Source: CAD feature listing. Evaluate the final solid. Frame: model axes, mm. Give positions to 0.01 mm unless a question says otherwise; leave off trailing zeros. Loops run counter-clockwise (first coordinate to the right, second up) from the corner with the lowest first, then second, coordinate; pieces in that order, holes last. Notation, with made-up numbers: (49.5, 5.5) -> (58.5, 5.5) arc R18 cw to (58.5, 36.5) -> close; hole circle Ø9 at (-25.75, -36). An arc over 180 degrees is marked (long way). Put each result on its own line as item: value.
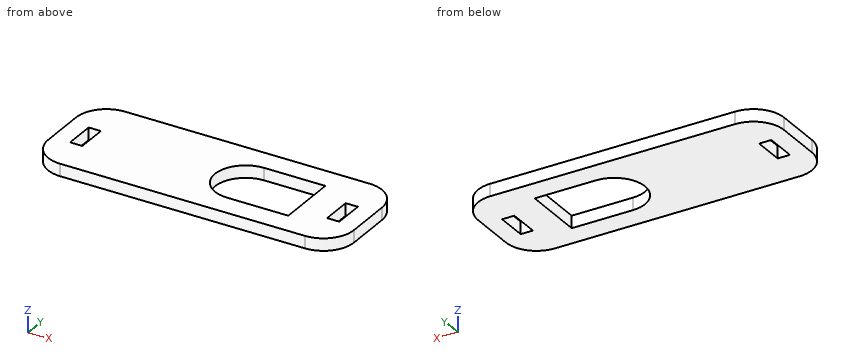
Autodesk Inventor part; units mm, degrees
ref_plane "YZ Plane" through (0, 0, 0) normal (1, 0, 0) x (0, 1, 0)
ref_plane "XZ Plane" through (0, 0, 0) normal (0, 1, 0) x (-1, 0, 0)
ref_plane "XY Plane" through (0, 0, 0) normal (0, 0, 1) x (1, 0, 0)
sketch "Эскиз1" plane through (0, 0, 0) normal (0, 0, 1) x (1, 0, 0)
  line L0 (40, -17.5) -> (22.4906, -17.5)
  arc A0 (40, -17.5) -> (50, -7.5) centre (40, -7.5) ccw
  line L1 (50, 7.5) -> (50, -7.5)
  arc A1 (50, 7.5) -> (40, 17.5) centre (40, 7.5) ccw
  line L2 (22.4906, 17.5) -> (40, 17.5)
  arc A2 (22.4906, 17.5) -> (53.3569, 60.2081) centre (-76.5583, 121.5932) ccw
  arc A3 (53.3569, 60.2081) -> (49.04, 63.7734) centre (57.3118, 69.3928) ccw
  arc A4 (49.04, 63.7734) -> (8.22, 17.5) centre (133.8701, -52.2004) ccw
  line L3 (-8.22, 17.5) -> (8.22, 17.5)
  arc A5 (-8.22, 17.5) -> (-49.04, 63.7734) centre (-133.8701, -52.2004) ccw
  arc A6 (-49.04, 63.7734) -> (-53.3569, 60.2081) centre (-57.3118, 69.3928) ccw
  arc A7 (-53.3569, 60.2081) -> (-22.4906, 17.5) centre (76.5583, 121.5932) ccw
  line L4 (-40, 17.5) -> (-22.4906, 17.5)
  arc A8 (-40, 17.5) -> (-50, 7.5) centre (-40, 7.5) ccw
  line L5 (-50, -7.5) -> (-50, 7.5)
  arc A9 (-50, -7.5) -> (-40, -17.5) centre (-40, -7.5) ccw
  line L6 (-22.4906, -17.5) -> (-40, -17.5)
  arc A10 (-22.4906, -17.5) -> (-53.3569, -60.2081) centre (76.5583, -121.5932) ccw
  arc A11 (-53.3569, -60.2081) -> (-49.04, -63.7734) centre (-57.3118, -69.3928) ccw
  arc A12 (-49.04, -63.7734) -> (-8.22, -17.5) centre (-133.8701, 52.2004) ccw
  line L7 (8.22, -17.5) -> (-8.22, -17.5)
  arc A13 (8.22, -17.5) -> (49.04, -63.7734) centre (133.8701, 52.2004) ccw
  arc A14 (49.04, -63.7734) -> (53.3569, -60.2081) centre (57.3118, -69.3928) ccw
  arc A15 (53.3569, -60.2081) -> (22.4906, -17.5) centre (-76.5583, -121.5932) ccw
  line L8 (22.4906, 17.5) -> (-22.4906, 17.5)
  line L9 (-22.4906, -17.5) -> (22.4906, -17.5)
  line L10 (25, 12.5) -> (25, 8.5)
  line L11 (25, 8.5) -> (15, 8.5)
  line L12 (15, 8.5) -> (15, 12.5)
  line L13 (15, 12.5) -> (25, 12.5)
  line L14 (-15, -8.5) -> (-15, -12.5)
  line L15 (-15, -12.5) -> (-25, -12.5)
  line L16 (-25, -12.5) -> (-25, -8.5)
  line L17 (-25, -8.5) -> (-15, -8.5)
  line L18 (25, -12.5) -> (15, -12.5)
  line L19 (15, -12.5) -> (15, -8.5)
  line L20 (15, -8.5) -> (25, -8.5)
  line L21 (25, -8.5) -> (25, -12.5)
  line L22 (-15, 8.5) -> (-25, 8.5)
  line L23 (-25, 8.5) -> (-25, 12.5)
  line L24 (-25, 12.5) -> (-15, 12.5)
  line L25 (-15, 12.5) -> (-15, 8.5)
  point P0 (0, 0)
  point P1 (8.22, 17.5)
  point P2 (-8.22, -17.5)
extrude "Выдавливание1" add sketch "Эскиз1" along normal blind 4 contours L0 L9 L7 L6 A9 L5 A8 L4 L8 L3 L2 A1 L1 A0 | L10 L11 L12 L13 | L14 L15 L16 L17 | L18 L19 L20 L21 | L22 L23 L24 L25
sketch "Эскиз3" plane through (0, 0, 0) normal (0, 0, -1) x (-1, 0, 0)
  point P0 (0, 0)
sketch "Эскиз4" plane through (0, 0, 0) normal (0, 0, -1) x (-1, 0, 0)
  point P0 (0, 0)
sketch "Эскиз5" plane through (0, 0, 0) normal (0, 0, -1) x (-1, 0, 0)
  line L0 (44, 4.453) -> (44, -5.547)
  line L1 (40, -5.547) -> (40, 4.453)
  line L2 (40, 4.453) -> (44, 4.453)
  line L3 (44, -5.547) -> (40, -5.547)
  line L4 (-44, -5.547) -> (-44, 4.453)
  line L5 (-40, 4.453) -> (-40, -5.547)
  line L6 (-44, 4.453) -> (-40, 4.453)
  line L7 (-40, -5.547) -> (-44, -5.547)
  line L8 (-10, 10) -> (-30, 10)
  line L9 (-30, 10) -> (-30, -10)
  line L10 (-30, -10) -> (-10, -10)
  line L11 (0, 0) -> (0, 0)
  arc A0 (0, 0) -> (-10, 10) centre (-10, 0) ccw
  arc A1 (-10, -10) -> (0, 0) centre (-10, 0) ccw
  point P0 (0, 0)
  point P1 (0, 10)
  dimension "d4" = 10
  dimension "d5" = 10
  dimension "d6" = 30
  dimension "d7" = 10
  dimension "d8" = 10
  dimension "d9" = 30
extrude "Выдавливание3" cut sketch "Эскиз5" against normal blind 4
sketch "Эскиз6" plane through (0, 0, 0) normal (0, 0, -1) x (-1, 0, 0)
  point P0 (0, 0)
properties part number "top"
(1) Line query: probe 1 along X at (y, z) = (-8, 2); probe 2 along X at (y, z) = (-1, 2.05); probe 3 along Y at (x, z) = (19, 0.25). Output: solid intervals per line, ascending. Write a range as from..to.
Calculated:
probe 1: x = -49.99..4, 30..49.99
probe 2: x = -50..-44, -40..0.05, 30..40, 44..50
probe 3: y = -17.5..-10, 10..17.5
(2) Section D-D on y = 6.5. Return loops of the section in (x, z), then the cut area to 3 significant figures.
Calculated:
outline: (-50, 0) -> (2.4, 0) -> (2.4, 4) -> (-50, 4) -> close; (30, 0) -> (50, 0) -> (50, 4) -> (30, 4) -> close
area: 290 mm²
(3) First-contact query: P1, Ø6, axis at x = 9, y = 5.5, coming from the -Z side; P2, Ø2, axis at x = -41.5, z = 2.5, coming from the +Y side; P3, Ø1.2, axis at x = 43, z = 2, coming from the -Y side; P4, Ø1.5, axis at y = 12, z = 1, coming from the +X side. Flat tips, straight axial feed; report the tip coordinate or a pass-through.
Calculated:
P1: passes through
P2: stops at y = 17.49
P3: stops at y = -17.21
P4: stops at x = 49.27
(4) Section C-C on z = 1.2. Return loops of the section in (x, y), then the cut area to 3 significant figures.
Calculated:
outline: (-50, -7.5) arc R10 ccw to (-40, -17.5) -> (40, -17.5) arc R10 ccw to (50, -7.5) -> (50, 7.5) arc R10 ccw to (40, 17.5) -> (-40, 17.5) arc R10 ccw to (-50, 7.5) -> close; hole (-44, -5.55) -> (-40, -5.55) -> (-40, 4.45) -> (-44, 4.45) -> close; hole (10, -10) -> (30, -10) -> (30, 10) -> (10, 10) arc R10 ccw to start; hole (40, -5.55) -> (44, -5.55) -> (44, 4.45) -> (40, 4.45) -> close
area: 2,780 mm²
(5) Section B-B on x = -42. Return loops of the section in (y, z), then the cut area to 3 significant figures.
Calculated:
outline: (-17.3, 0) -> (-5.55, 0) -> (-5.55, 4) -> (-17.3, 4) -> close; (4.45, 0) -> (17.3, 0) -> (17.3, 4) -> (4.45, 4) -> close
area: 98.4 mm²
(6) Section A-A on y = 0. Return loops of the section in (x, z), then the cut area to 3 significant figures.
Calculated:
outline: (-50, 0) -> (-44, 0) -> (-44, 4) -> (-50, 4) -> close; (-40, 0) -> (0, 0) -> (0, 4) -> (-40, 4) -> close; (30, 0) -> (40, 0) -> (40, 4) -> (30, 4) -> close; (44, 0) -> (50, 0) -> (50, 4) -> (44, 4) -> close
area: 248 mm²
